Autodesk Inventor part; units mm, degrees
ref_plane "РабПлоскость1" through (0, 0, 75.2) normal (0, 0, 1) x (1, 0, 0)
ref_plane "YZ Plane" through (0, 0, 0) normal (1, 0, 0) x (0, 1, 0)
ref_plane "XZ Plane" through (0, 0, 0) normal (0, 1, 0) x (-1, 0, 0)
ref_plane "РабПлоскость1" through (0, 0, 75.2) normal (0, 0, 1) x (1, 0, 0)
sketch "Эскиз1" plane through (0, 0, 75.2) normal (0, 0, 1) x (1, 0, 0)
  circle A0 centre (26.4645, -26.4645) radius 1.95 construction
  circle A1 centre (-26.4645, 26.4645) radius 1.95 construction
  circle A2 centre (26.4645, 26.4645) radius 1.95 construction
  circle A3 centre (-26.4645, -26.4645) radius 1.95 construction
  circle A4 centre (15.35, -15.35) radius 1.7 construction
  circle A5 centre (-15.35, 15.35) radius 1.7 construction
  circle A6 centre (15.35, 15.35) radius 1.7 construction
  circle A7 centre (-15.35, -15.35) radius 1.7 construction
  line L0 (-32.5, 27.5) -> (-32.5, -27.5)
  line L1 (-27.5, 32.5) -> (-32.5, 27.5)
  line L2 (27.5, 32.5) -> (-27.5, 32.5)
  line L3 (32.5, 27.5) -> (27.5, 32.5)
  line L4 (32.5, -27.5) -> (32.5, 27.5)
  line L5 (27.5, -32.5) -> (32.5, -27.5)
  line L6 (-27.5, -32.5) -> (27.5, -32.5)
  line L7 (-32.5, -27.5) -> (-27.5, -32.5)
  circle A8 centre (0, 0) radius 11.5 construction
  circle A9 centre (0, 0) radius 26.7
  point P0 (0, 0)
extrude "Выдавливание1" add sketch "Эскиз1" along normal blind 4
sketch "Эскиз2" plane through (0, 0, 79.2) normal (0, 0, 1) x (1, 0, 0)
  circle A0 centre (26.4645, 26.4645) radius 2.25
  circle A1 centre (26.4645, -26.4645) radius 2.25
  circle A2 centre (-26.4645, -26.4645) radius 2.25
  circle A3 centre (-26.4645, 26.4645) radius 1.95
  circle A4 centre (10.5, 29.5) radius 2.25 construction
  circle A5 centre (-10.5, 29.5) radius 1.65 construction
hole "Отверстие1" at (26.4645, 26.4645, 79.2) at (-26.4645, 26.4645, 79.2) at (26.4645, -26.4645, 79.2) at (-26.4645, -26.4645, 79.2) at (10.5, 29.5, 79.2) at (-10.5, 29.5, 79.2) direction (0, 0, -1) diameter 3.4 end through all countersink diameter 6 countersink angle 90
sketch "Эскиз3" plane through (0, 0, 75.2) normal (0, 0, -1) x (-1, 0, 0)
  line L0 (-21.5, 32.5) -> (-13.5, 32.5) construction
  line L1 (-13.5, 32.5) -> (-13.5, 22.5) construction
  line L2 (-13.5, 22.5) -> (-21.5, 22.5) construction
  line L3 (-21.5, 22.5) -> (-21.5, 32.5) construction
  line L4 (13.5, 32.5) -> (21.5, 32.5) construction
  line L5 (21.5, 32.5) -> (21.5, 22.5) construction
  line L6 (21.5, 22.5) -> (13.5, 22.5) construction
  line L7 (13.5, 22.5) -> (13.5, 32.5) construction
  line L8 (0, 0) -> (0, 42.6658) construction
  line L9 (-27.5, 32.5) -> (27.5, 32.5) construction
  line L10 (-21.3, 32.5) -> (-13.7, 32.5)
  line L11 (-13.7, 32.5) -> (-13.7, 23.5)
  line L12 (-13.7, 23.5) -> (-21.3, 23.5)
  line L13 (-21.3, 23.5) -> (-21.3, 32.5)
  line L14 (13.7, 32.5) -> (21.3, 32.5)
  line L15 (21.3, 32.5) -> (21.3, 23.5)
  line L16 (21.3, 23.5) -> (13.7, 23.5)
  line L17 (13.7, 23.5) -> (13.7, 32.5)
  dimension "d9" = 10
  dimension "d10" = 0.2
  dimension "d11" = 0.2
  dimension "d12" = 9
extrude "Выдавливание2" add sketch "Эскиз3" along normal blind 12
sketch "Эскиз4" plane through (-27.5, 32.5, 79.2) normal (0, 1, 0) x (1, 0, 0)
  arc A0 (14, 16) -> (6, 16) centre (10, 16) ccw
  arc A1 (49, 16) -> (41, 16) centre (45, 16) ccw
  circle A2 centre (45, 16) radius 4
  circle A3 centre (10, 16) radius 4
  point P0 (27.5, 79.2)
extrude "Выдавливание3" cut sketch "Эскиз4" against normal through all
fillet "Сопряжение1" radius 0.2 4 edges at (-21.3, 28, 64.449) (-13.7, 28, 64.449) (13.7, 28, 64.449) (21.3, 28, 64.449)
sketch "Эскиз5" plane through (0, 0, 75.2) normal (0, 0, -1) x (-1, 0, 0)
  line L0 (14.0714, 23.5) -> (14.0714, 32.5) construction
  line L1 (20.9286, 23.5) -> (14.0714, 23.5) construction
  line L2 (20.9286, 32.5) -> (20.9286, 23.5) construction
  line L3 (14.0714, 32.5) -> (20.9286, 32.5) construction
  line L4 (-20.9286, 23.5) -> (-20.9286, 32.5) construction
  line L5 (-14.0714, 23.5) -> (-20.9286, 23.5) construction
  line L6 (-14.0714, 32.5) -> (-14.0714, 23.5) construction
  line L7 (-20.9286, 32.5) -> (-14.0714, 32.5) construction
  line L8 (20.9286, 23.5) -> (14.0714, 32.5) construction
  line L9 (19, 32.5) -> (16, 32.5)
  line L10 (16, 32.5) -> (16, 23.5)
  line L11 (16, 23.5) -> (19, 23.5)
  line L12 (19, 23.5) -> (19, 32.5)
  line L13 (19, 32.5) -> (16, 23.5) construction
  line L14 (16, 32.5) -> (19, 23.5) construction
  point P0 (0, 0)
  point P1 (17.5, 28)
  dimension "d18" = 3
extrude "Выдавливание4" add sketch "Эскиз5" along normal blind 9
mirror "Зеркальное отражение1" about plane through (0, 0, 0) normal (1, 0, 0) of "Выдавливание4"
equation "\"d11\" = d10"
properties part number "Крышка" material "По умолчанию1"
Source: CAD feature listing. Evaluate the final solid. Frame: model axes, mm. A direction names the side the tool comes from. Coordinates: 2 decimals unless noted, no trailing zeros. Loops run counter-clockwise (first coordinate to the right, second up) from the corner with the lowest first, then second, coordinate; pieces in that order, holes last. Notation, with made-up numbers: (-5, 53) - (34, 53) arc R20 cw to (34, 76) - close; hole circle Ø3 at (17, 11.5). An arc over 180 degrees is marked (long way). One line per item, written item: value. Start each with the question number.
1. Contact query for flat-ended pins moving along their axis: P1, Ø2.5, axis at y = 26, z = 72, coming from the -X side; P2, Ø4, axis at x = -26.46, y = 26.46, coming from the -Z side; P3, Ø2.5, axis at x = 17, y = 28, coming from the -Z side; P4, Ø8, axis at x = 23.5, y = -2, coming from the +Z side. Output: stop coordinate, or through.
2. Section B-B (z = 69.75). Return the cut outline in (x, y).
3. Set-up query: faces 1 (the cylindrical face through (-9.85, 27.93, 76.53)), 2 (the flat face through (18, 28, 66.2)). Return all of +Z, -Z, +X, -X, +Y, -Y with unobstructed straight access to the full face (end or side cutting, diameter ignored); none if empty.
4. Mould query, pull axis X, two halves, no side actions, for faces 3 (the flat face through (-17, 23.5, 70)), 4 (the flat face through (-32.5, 0, 77)), 5 (the cylindrical face through (25.467, -8.02, 77.172)). Classes: pulls with the +X half, pulls with the -X half, needs draft (parallel to the pull), parting line crosses it, or undercut.
5. Ray query, L1, parallel to X at y = 25, z = 72.75; L2, parallel to X at y = 29.5, z = 76.6; L3, parallel to Y at x = 19, z = 67.25. Return the intervals inside material, ascending.
6. Section A-A (y = 0). Return the cut outline in (x, z).
Verdict:
1. P1: stops at x = -21.3
1. P2: stops at z = 75.2
1. P3: stops at z = 66.2
1. P4: stops at z = 79.2
2. outline: (-21.3, 23.5) - (-13.7, 23.5) - (-13.7, 32.5) - (-21.3, 32.5) - close; (13.7, 23.5) - (21.3, 23.5) - (21.3, 32.5) - (13.7, 32.5) - close
3. face 1: +Z, -Z
3. face 2: -Z, +Y, -Y
4. face 3: needs draft
4. face 4: pulls with the -X half
4. face 5: undercut
5. L1: x = -21.3 to -13.7, 13.7 to 21.3
5. L2: x = -30.5 to -12.2, -8.8 to 8.8, 12.2 to 30.5
5. L3: y = 23.5 to 32.5
6. outline: (-32.5, 75.2) - (-26.7, 75.2) - (-26.7, 79.2) - (-32.5, 79.2) - close; (26.7, 75.2) - (32.5, 75.2) - (32.5, 79.2) - (26.7, 79.2) - close
